Design review of the part shown in the three views and the two pictorial views. Dimensions are in mm from the part's minimum x, y and z. A direction names the side the tool comes from. Give positions to 0.01 mm unless a question says otherwise; leave off trailing zeros. Order: outer loops, then holes, each group sorted by start corner. A loop starts at its lowest first (then second) coordinate and runs counter-clockwise, first axis right, second up. Notation, with made-up numbers: (-12, 57) - (13, 57) arc R24 ccw to (13, 78) - close; hole circle Ø2 at (-29.5, 41.25). An arc over 180 degrees is marked (long way). Put each result on its own line as item: value. Start each with the question number.
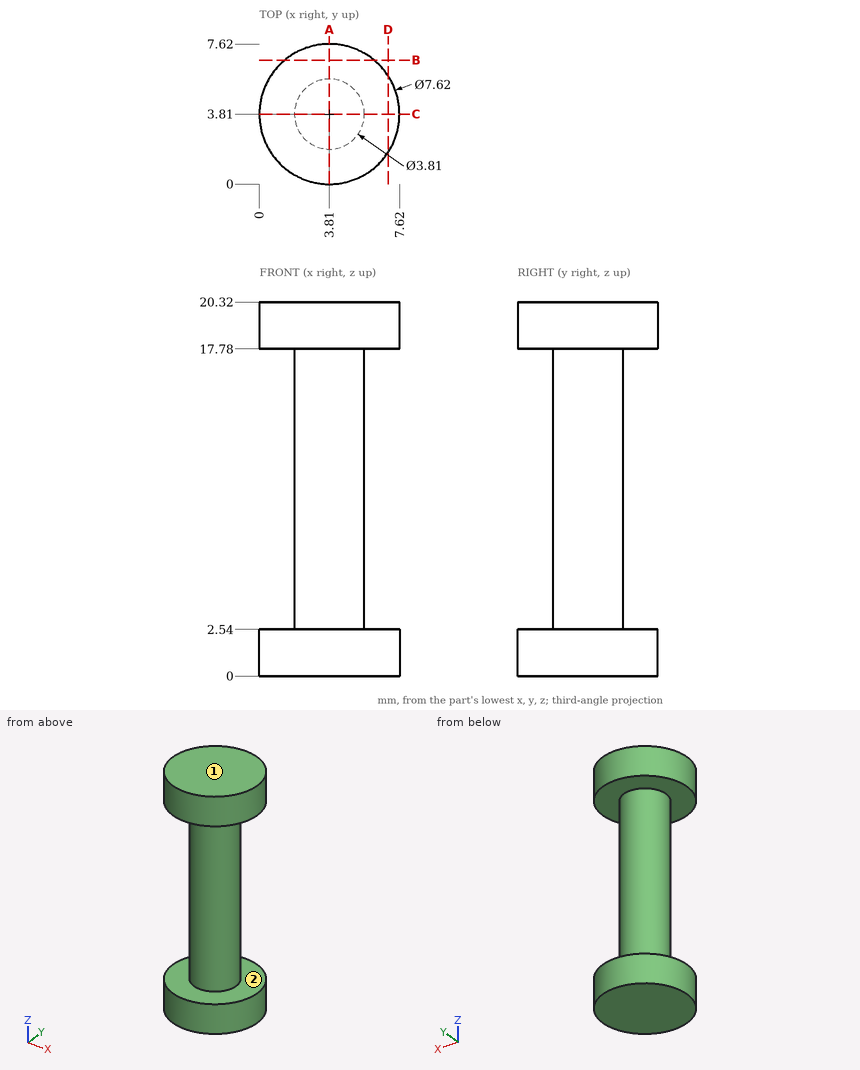
1. Add section A-A, the plane x = 3.81. Give the boundary of the cut face in (y, z) (3 decimals), then the cut area to 3 significant figures.
2. Add section B-B, the plane y = 6.75. Give the boundary of the cut face in (x, z).
3. Tool access review of the marked faces 1 and 2: name each direction out of +Z, -Z, +X, -X, +Y, -Y from which nothing blocks a thin tool from reaching the whole face with its end or side.
4. Wall thickness on line 1 (Z direction, x = 5.75, y = 5); line 2 (X direction, y = 5.5, z = 16): over which ranges is each line inside the solid? List them lowest first. Write a range as from..to.
5. Clearance check with a flat-ended pin moving along its axis: pin 1 (1.5 mm diameter, centred on x = 1, z = 7, fed in from -Y). State where the tip first meets the part, or that it passes through.
6. Add section D-D, the plane x = 7. Give the boundary of the cut face in (y, z), then the cut area to 3 significant figures.
Found:
1. outline: (0, 0) - (7.62, 0) - (7.62, 2.54) - (5.715, 2.54) - (5.715, 17.78) - (7.62, 17.78) - (7.62, 20.32) - (0, 20.32) - (0, 17.78) - (1.905, 17.78) - (1.905, 2.54) - (0, 2.54) - close
1. area: 96.8 mm^2
2. outline: (1.39, 0) - (6.23, 0) - (6.23, 2.54) - (1.39, 2.54) - close; (1.39, 17.78) - (6.23, 17.78) - (6.23, 20.32) - (1.39, 20.32) - close
3. face 1: +Z, +X, -X, +Y, -Y
3. face 2: none
4. line 1: z = 0..2.54, 17.78..20.32
4. line 2: x = 2.93..4.69
5. pin 1: passes through
6. outline: (1.73, 0) - (5.89, 0) - (5.89, 2.54) - (1.73, 2.54) - close; (1.73, 17.78) - (5.89, 17.78) - (5.89, 20.32) - (1.73, 20.32) - close
6. area: 21.2 mm^2
